Could you check a few things on this model? Use its own coordinates, in mm. A direction names the side the tool comes from. Coordinates: 2 decimals unless noted, no trailing zeros. Order: outer loops, then holes, each group sorted by start corner. A loop starts at its lowest first (then second) coordinate and runs counter-clockwise, first axis right, second up. Notation, with made-up numbers: M 67,66 L 116,66 A19 cw 116,79 Z; hole C 46.25,88.25 d6. An arc over 180 degrees is marked long. Write item = value, one per line. Start each with the question number.
Autodesk Inventor part; units mm, degrees
ref_plane "YZ Plane" through (0, 0, 0) normal (1, 0, 0) x (0, 1, 0)
ref_plane "XZ Plane" through (0, 0, 0) normal (0, 1, 0) x (-1, 0, 0)
ref_plane "XY Plane" through (0, 0, 0) normal (0, 0, 1) x (1, 0, 0)
sketch "スケッチ1" plane through (0, 0, 0) normal (0, 1, 0) x (-1, 0, 0)
  line L0 (0, 0) -> (-38, 0)
  line L1 (-38, 0) -> (-38, -44)
  line L2 (-38, -44) -> (0, -44)
  line L3 (0, -44) -> (0, 0)
  dimension "d0" = 44
  dimension "d1" = 38
extrude "押し出し1" add sketch "スケッチ1" along normal blind 39.5
sketch "スケッチ2" plane through (38, 0, -44) normal (0, 0, -1) x (-1, 0, 0)
  line L0 (3, 36.5) -> (59.072, 36.5)
  line L1 (59.072, 36.5) -> (59.072, 3)
  line L2 (59.072, 3) -> (3, 3)
  line L3 (3, 3) -> (3, 36.5)
  line L4 (0, 39.5) -> (38, 39.5)
  line L5 (0, 0) -> (38, 0)
  line L6 (0, 0) -> (0, 39.5)
  dimension "d4" = 33.5
  dimension "d6" = 3
  dimension "d7" = 3
extrude "押し出し2" cut sketch "スケッチ2" against normal blind 100
sketch "スケッチ3" plane through (0, 39.5, 0) normal (0, 1, 0) x (1, 0, 0)
  line L0 (38, 44) -> (0, 44)
  line L1 (38, 0) -> (38, 44)
  point P0 (0, 0)
  point P1 (17, 28)
  dimension "d10" = 16
  dimension "d11" = 21
hole "穴1" at (17, 39.5, -28) direction (0, -1, 0) diameter 22 end through all
sketch "スケッチ4" plane through (0, 39.5, 0) normal (0, 1, 0) x (1, 0, 0)
  line L0 (0, 0) -> (38, 0)
  line L1 (38, 0) -> (38, 44)
  point P0 (30.5, 4)
  point P1 (30.5, 31)
  point P2 (3.5, 4)
  point P3 (3.5, 31)
  point P4 (3.5, 4)
  dimension "d19" = 4
  dimension "d20" = 7.5
  dimension "d23" = 27
  dimension "d26" = 27
hole "穴2" at (30.5, 39.5, -4) at (30.5, 39.5, -31) at (3.5, 39.5, -31) at (3.5, 39.5, -4) direction (0, -1, 0) diameter 3.2 end through all
fillet "フィレット1" radius 2 2 edges at (35, 3, -22) (35, 36.5, -22)
sketch "スケッチ7" plane through (0, 39.5, 0) normal (0, 1, 0) x (1, 0, 0)
  line L0 (38, 44) -> (0, 44)
  line L1 (6, 44) -> (28, 44)
  line L2 (28, 44) -> (28, 28)
  line L3 (28, 28) -> (6, 28)
  line L4 (6, 28) -> (6, 44)
  circle A0 centre (17, 28) radius 11
  point P0 (0, 0)
  point P1 (28, 28)
  point P2 (28, 44)
  dimension "d69" = 22
  dimension "d70" = 11
  dimension "d84" = 0
extrude "押し出し3" cut sketch "スケッチ7" against normal through all contours L2 A0 L4 L0
sketch "スケッチ8" plane through (35, 5, -44) normal (-1, 0, 0) x (0, 0, 1)
  line L0 (12, 4.5) -> (34, 4.5)
  line L1 (34, 4.5) -> (34, 19.5)
  line L2 (34, 19.5) -> (12, 19.5)
  line L3 (12, 19.5) -> (12, 4.5)
  line L4 (44, 34.5) -> (44, 0)
  line L5 (44, 34.5) -> (0, 34.5)
  point P0 (44, -5)
  point P1 (44, 29.5)
  dimension "d73" = 10
  dimension "d74" = 22
  dimension "d75" = 15
  dimension "d76" = 15
hole "穴5" at (35, 9.5, -10) at (35, 9.5, -32) at (35, 24.5, -32) at (35, 24.5, -10) direction (1, 0, 0) diameter 2.5 end through all
properties part number "サーボモータ固定用２軸目3mm改_printer"
(1) Will these pins go through, and if not, where does the flat tip stop? P1, Ø4, axis at y = 9.5, z = -32, coming from the -X side; P2, Ø6, axis at y = 6.5, z = -39, coming from the -X side; P3, Ø1.5, axis at y = 34.5, z = -6, coming from the -X side.
(2) Thinking about a two-plate mould opening in Z: for faces 1 (the cylindrical face through (2.42, 37.98, -32.18)), 2 (the cylindrical face through (2.42, 1.48, -32.18)), 3 (the cylindrical face through (34.43, 35.9, -21.69)), 4 (the cylindrical face through (17, 38, -17)), which applies, released by +Z, released by -Z, zero draft, split by the parting line, or undercut?
(3) Imagine slicing it at B-B on z = -4. List the corners of the cut face in (x, y) for me.
(4) Imagine slicing it at A-A on x = 17. List the corners of the cut face in (y, z) for me, plus the area to 3 significant figures.
(5) Please list where these lines run through material, in increasing order: probe 1 along Y at (x, z) = (37.2, -32); probe 2 along X at (y, z) = (2, -31); probe 3 along X at (y, z) = (0.9, -4). Write a range as from..to.
(6) Imagine slicing it at C-C on x = 30.5. List the corners of the cut face in (y, z) for me, plus the area to 3 significant figures.
(7) Imagine slicing it at D-D on y = 24.5. List the corners of the cut face in (x, z) for me, plus the area to 3 significant figures.
(8) For faces 5 (the flat face through (28, 38, -36)), 6 (the flat face through (35, 20, -22)), 7 (the flat face through (19, 0, -17)), which set-ups out of +Z, -Z, +X, -X, +Y, -Y let a thin tool reach every point of the face, with its end or its side?
Response:
q1.P1 = 35
q1.P2 = 34.32
q1.P3 = 34.85
q2.face_1 = undercut
q2.face_2 = undercut
q2.face_3 = zero draft
q2.face_4 = released by -Z
q3.outline = M 0,0 L 1.9,0 L 1.9,3 L 0,3 Z; M 0,36.5 L 1.9,36.5 L 1.9,39.5 L 0,39.5 Z; M 5.1,0 L 28.9,0 L 28.9,3 L 5.1,3 Z; M 5.1,36.5 L 28.9,36.5 L 28.9,39.5 L 5.1,39.5 Z; M 32.1,0 L 38,0 L 38,39.5 L 32.1,39.5 L 32.1,36.5 L 33,36.5 A2 cw 35,34.5 L 35,5 A2 cw 33,3 L 32.1,3 Z
q4.outline = M 0,-17 L 3,-17 L 3,0 L 0,0 Z; M 36.5,-17 L 39.5,-17 L 39.5,0 L 36.5,0 Z
q4.area = 102 mm2
q5.probe_1 = 0..8.25, 10.75..23.25, 25.75..39.5
q5.probe_2 = 0..1.9, 5.1..6, 28..28.9, 32.1..38
q5.probe_3 = 0..1.9, 5.1..28.9, 32.1..38
q6.outline = M 0,-44 L 3,-44 L 3,-32.6 L 0,-32.6 Z; M 0,-29.4 L 3,-29.4 L 3,-5.6 L 0,-5.6 Z; M 0,-2.4 L 3,-2.4 L 3,0 L 0,0 Z; M 36.5,-44 L 39.5,-44 L 39.5,-32.6 L 36.5,-32.6 Z; M 36.5,-29.4 L 39.5,-29.4 L 39.5,-5.6 L 36.5,-5.6 Z; M 36.5,-2.4 L 39.5,-2.4 L 39.5,0 L 36.5,0 Z
q6.area = 226 mm2
q7.outline = M 35,-44 L 38,-44 L 38,-33.25 L 35,-33.25 Z; M 35,-30.75 L 38,-30.75 L 38,-11.25 L 35,-11.25 Z; M 35,-8.75 L 38,-8.75 L 38,0 L 35,0 Z
q7.area = 117 mm2
q8.face_5 = -Z, +Y, -Y
q8.face_6 = +Z, -Z, -X
q8.face_7 = +Z, -Z, +X, -X, -Y
